Autodesk Inventor part; units mm, degrees
ref_plane "YZ Plane" through (0, 0, 0) normal (1, 0, 0) x (0, 1, 0)
ref_plane "XZ Plane" through (0, 0, 0) normal (0, 1, 0) x (-1, 0, 0)
ref_plane "XY Plane" through (0, 0, 0) normal (0, 0, 1) x (1, 0, 0)
sketch "Szkic1" plane through (0, 0, 0) normal (0, 0, 1) x (1, 0, 0)
  line L0 (-172.0995, -130.735) -> (1627.9005, -130.735)
  line L1 (1627.9005, -130.735) -> (1627.9005, -330.735)
  line L2 (1627.9005, -330.735) -> (-172.0995, -330.735)
  line L3 (-172.0995, -330.735) -> (-172.0995, -130.735)
  dimension "d6" = 1800
  dimension "d7" = 200
extrude "Wyciągnięcie proste1" add sketch "Szkic1" along normal blind 1100
sketch "Szkic2" plane through (-172.0995, -130.735, 0) normal (0, 1, 0) x (1, 0, 0)
  point P0 (172.0995, 0)
sketch "Szkic3" plane through (-172.0995, -130.735, 0) normal (0, 1, 0) x (1, 0, 0)
  line L0 (0, 0) -> (1800, 0)
  line L1 (0, -1100) -> (1800, -1100)
  line L2 (0, 0) -> (200, 0)
  line L3 (200, 0) -> (200, -1100)
  line L4 (200, -1100) -> (0, -1100)
  line L5 (0, -1100) -> (0, 0)
  line L6 (1800, 0) -> (1700, 0)
  line L7 (1700, -1100) -> (1800, -1100)
  line L8 (1334, 0) -> (1134, 0)
  line L9 (1134, 0) -> (1134, -1100)
  line L10 (1134, -1100) -> (1334, -1100)
  line L11 (1334, -1100) -> (1334, 0)
  line L12 (100, 0) -> (100, -1100)
  line L13 (1234, 0) -> (1234, -1100) construction
  point P0 (172.0995, 0)
  point P1 (1134, 0)
  dimension "d10" = 200
  dimension "d15" = 200
  dimension "d21" = 934
extrude "Wyciągnięcie proste2" add sketch "Szkic3" along normal blind 1200 contours L0 L12 L1 L5 | L0 L3 L1 L12 | L0 L11 L1 L9
sketch "Szkic6" plane through (27.9005, -130.735, 1100) normal (1, 0, 0) x (0, 0, -1)
  line L0 (0, 1200) -> (1100, 1200)
  line L1 (550, 1200) -> (550, 0)
  line L2 (1100, 0) -> (0, 0)
  line L3 (0, 0) -> (0, 1200)
  line L4 (0, 600) -> (1100, 600)
  line L5 (1100, 0) -> (1100, 1200)
  circle A0 centre (550, 600) radius 85
  point P0 (1100, 130.735)
  dimension "d23" = 170
extrude "Wyciągnięcie proste4" cut sketch "Szkic6" along normal blind 982 and the other way blind 46 contours A0 L4 L1 | L1 L4 A0 | L4 L1 A0 | L4 A0 L1
sketch "Szkic7" plane through (1161.9005, -130.735, 1100) normal (1, 0, 0) x (0, 0, -1)
  point P0 (1100, 130.735)
sketch "Szkic8" plane through (1161.9005, -130.735, 1100) normal (1, 0, 0) x (0, 0, -1)
  circle A0 centre (550, 600) radius 85
  circle A1 centre (550, 600) radius 132
  point P0 (1100, 130.735)
  dimension "d28" = 264
extrude "Wyciągnięcie proste5" cut sketch "Szkic8" against normal up to surface (152 mm away) contours A0 | A1
sketch "Szkic9" plane through (-172.0995, -330.735, 0) normal (-1, 0, 0) x (0, 0, 1)
  circle A0 centre (550, 800) radius 85
  circle A1 centre (550, 800) radius 132
  point P0 (0, 330.735)
extrude "Wyciągnięcie proste6" cut sketch "Szkic9" against normal up to surface (154 mm away) contours A0 | A1
sketch "Szkic10" plane through (1161.9005, -130.735, 1100) normal (1, 0, 0) x (0, 0, -1)
  line L0 (1100, 1200) -> (0, 1200)
  line L1 (1100, 0) -> (0, 0)
  line L2 (0, -200) -> (0, 1200)
  circle A0 centre (550, 600) radius 250
  line L3 (0, 0) -> (322.7328, 704.1616)
  line L4 (1100, 0) -> (777.2672, 704.1616)
  line L5 (0, 0) -> (0, 1200)
  line L6 (0, 1200) -> (1100, 1200)
  line L7 (1100, -200) -> (1100, 1200)
  line L8 (1100, 1200) -> (1100, 0)
  point P0 (1100, 130.735)
  dimension "d33" = 500
extrude "Wyciągnięcie proste7" cut sketch "Szkic10" against normal through all contours L7 L4 A0 L3 L2 L0
sketch "Szkic11" plane through (-172.0995, -330.735, 0) normal (-1, 0, 0) x (0, 0, 1)
  circle A0 centre (550, 800) radius 132
  circle A1 centre (550, 800) radius 85
  circle A2 centre (550, 800) radius 250
  line L0 (0, 200) -> (1100, 200)
  line L1 (0, 0) -> (1100, 0)
  line L2 (1100, 0) -> (1100, 200)
  line L3 (1100, 200) -> (0, 200)
  line L4 (0, 200) -> (0, 0)
  line L5 (1100, 200) -> (777.2672, 904.1616)
  line L6 (1100, 200) -> (777.2672, 904.1616)
  line L7 (322.7328, 904.1616) -> (0, 200)
  line L8 (0, 200) -> (322.7328, 904.1616)
  point P0 (0, 330.735)
extrude "Wyciągnięcie proste8" add sketch "Szkic11" along normal blind 48 contours A2 | A2 L5 L0 L7 | L2 L1 L4 L0
sketch "Szkic12" plane through (-220.0995, -330.735, 0) normal (-1, 0, 0) x (0, 0, 1)
  point P0 (0, 330.735)
sketch "Szkic13" plane through (-18.0995, 469.265, 550) normal (-1, 0, 0) x (0, 0, 1)
  point P0 (-550, -469.265)
ref_plane "Płaszczyzna konstrukcyjna1" through (-220.0995, -330.735, 0) normal (-1, 0, 0) x (0, 0, 1)
sketch "Szkic14" plane through (-220.0995, -330.735, 0) normal (-1, 0, 0) x (0, 0, 1)
  point P0 (0, 330.735)
sketch "Szkic15" plane through (-220.0995, -330.735, 0) normal (-1, 0, 0) x (0, 0, 1)
  point P0 (0, 330.735)
sketch "Szkic16" plane through (-220.0995, -330.735, 0) normal (-1, 0, 0) x (0, 0, 1)
  circle A0 centre (550, 980) radius 18
  point P0 (0, 330.735)
  dimension "d39" = 36
extrude "Wyciągnięcie proste9" cut sketch "Szkic16" against normal blind 35
sketch "Szkic18" plane through (-220.0995, -330.735, 0) normal (-1, 0, 0) x (0, 0, 1)
  circle A0 centre (550, 620) radius 18
  circle A1 centre (370, 800) radius 18
  point P0 (0, 330.735)
  dimension "d43" = 36
  dimension "d44" = 36
extrude "Wyciągnięcie proste10" cut sketch "Szkic18" against normal blind 35
thread "Gwint1"
thread "Gwint2"
thread "Gwint3"
sketch "Szkic19" plane through (-220.0995, -330.735, 0) normal (-1, 0, 0) x (0, 0, 1)
  circle A0 centre (730, 800) radius 18
  point P0 (0, 330.735)
  dimension "d57" = 36
extrude "Wyciągnięcie proste12" cut sketch "Szkic19" against normal blind 35
thread "Gwint5"
sketch "Szkic20" plane through (27.9005, -130.735, 1100) normal (1, 0, 0) x (0, 0, -1)
  point P0 (1100, 130.735)
sketch "Szkic26" plane through (961.9005, -130.735, 0) normal (-1, 0, 0) x (0, 0, 1)
  circle A0 centre (550, 600) radius 85
  circle A1 centre (550, 600) radius 250
  point P0 (0, 130.735)
extrude "Wyciągnięcie proste15" add sketch "Szkic26" along normal blind 126
sketch "Szkic27" plane through (835.9005, 469.265, 550) normal (-1, 0, 0) x (0, 0, 1)
  circle A0 centre (0, 0) radius 87
  circle A1 centre (0, 0) radius 92
  point P0 (-550, -469.265)
  dimension "d71" = 174
  dimension "d72" = 184
extrude "Wyciągnięcie proste16" cut sketch "Szkic27" against normal blind 8
sketch "Szkic28" plane through (-220.0995, -330.735, 0) normal (-1, 0, 0) x (0, 0, 1)
  point P0 (0, 330.735)
sketch "Szkic29" plane through (1161.9005, -130.735, 1100) normal (1, 0, 0) x (0, 0, -1)
  circle A0 centre (550, 780) radius 18
  circle A1 centre (550, 780) radius 18
  circle A2 centre (730, 600) radius 18
  circle A3 centre (730, 600) radius 18
  circle A4 centre (550, 420) radius 18
  circle A5 centre (550, 420) radius 18
  circle A6 centre (370, 600) radius 18
  circle A7 centre (370, 600) radius 18
  point P0 (1100, 130.735)
  dimension "d75" = 36
  dimension "d76" = 36
  dimension "d77" = 36
  dimension "d78" = 36
extrude "Wyciągnięcie proste17" cut sketch "Szkic29" against normal blind 35
thread "Gwint6"
thread "Gwint7"
thread "Gwint8"
thread "Gwint9"
sketch "Szkic30" plane through (27.9005, -130.735, 1100) normal (1, 0, 0) x (0, 0, -1)
  circle A0 centre (550, 600) radius 250
  point P0 (1100, 130.735)
  dimension "d89" = 500
extrude "Wyciągnięcie proste18" add sketch "Szkic30" along normal blind 126
sketch "Szkic31" plane through (153.9005, 469.265, 550) normal (1, 0, 0) x (0, 0, -1)
  point P0 (550, -469.265)
sketch "Szkic32" plane through (153.9005, 469.265, 550) normal (1, 0, 0) x (0, 0, -1)
  circle A0 centre (0, 0) radius 85
  circle A1 centre (0, 0) radius 85
  point P0 (550, -469.265)
  dimension "d92" = 170
extrude "Wyciągnięcie proste19" cut sketch "Szkic32" against normal blind 400
sketch "Szkic33" plane through (153.9005, 469.265, 550) normal (1, 0, 0) x (0, 0, -1)
  circle A0 centre (0, 0) radius 87
  circle A1 centre (0, 0) radius 92
  point P0 (550, -469.265)
  dimension "d95" = 174
  dimension "d96" = 184
extrude "Wyciągnięcie proste20" cut sketch "Szkic33" against normal blind 8
properties part number "podstawa"
Check sheet for the modelled part. Datum: model origin and axes. Units: mm. A direction names the side the tool comes from. Coordinates: 2 decimals unless noted, no trailing zeros. Loops run counter-clockwise (first coordinate to the right, second up) from the corner with the lowest first, then second, coordinate; pieces in that order, holes last. Notation, with made-up numbers: (33.25, 33.25) -> (76.25, 33.25) arc R18 ccw to (76.25, 44.25) -> close; hole circle Ø7 at (-10.5, -18). An arc over 180 degrees is marked (long way). Answer in a Markdown table with one row per item.
1. Sectioned sample at A-A, the plane y = 24. Record the boundary of the cut face in (x, z), then the cut area to 3 significant figures.
Check values:
| item | result |
|---|---|
| outline | (-220.1, 70.92) -> (27.9, 70.92) -> (27.9, 1029.08) -> (-220.1, 1029.08) -> close; (961.9, 70.92) -> (1161.9, 70.92) -> (1161.9, 1029.08) -> (961.9, 1029.08) -> close |
| area | 429,000 mm2 |
2. Release check for a two-part mould opening along Y. For faces 1 (the face through (149.956, 413.284, 623.008)), 2 (the face through (1161.9, 194, 558)), 3 (the face through (717, -330.735, 542)) record: released by +Y, released by -Y, zero draft, split by the parting line, or undercut.
Check values:
| item | result |
|---|---|
| face 1 | undercut |
| face 2 | zero draft |
| face 3 | released by -Y |
3. Go/stop test with flat-tipped pins: pin 1 (11 mm diameter, centred on y = 645, z = 548, fed in from +X); pin 2 (5 mm diameter, centred on y = 585, z = 595.5, fed in from +X); pin 3 (1.5 mm diameter, centred on x = -6.5, z = 701.5, fed in from +Y). Record where each tip stops, or that it passes through.
Check values:
| item | result |
|---|---|
| pin 1 | stops at x = 1126.9 |
| pin 2 | stops at x = 1009.9 |
| pin 3 | stops at y = 668.7 |
4. Material ranges on line 1 along Y through (x, z) = (-196, 550) (3 decimals); line 2 along Y through (x, z) = (1124.5, 550) (3 decimals); line 3 along X through (y, z) = (529, 696), recorded low to high. Write a range as [from, to].
Check values:
| item | result |
|---|---|
| line 1 | y = [-330.735, 271.265], [307.265, 337.265], [601.265, 631.265], [667.265, 719.265] |
| line 2 | y = [-330.735, 337.265], [601.265, 719.265] |
| line 3 | x = [-220.1, 153.9], [835.9, 1161.9] |
5. Sectioned sample at B-B, the plane z = 499. Give the number of separate pieces and of enclosed holes in the cut face, then the cut area to 3 significant figures.
Check values:
| item | result |
|---|---|
| separate pieces | 3 |
| enclosed holes | 0 |
| area | 738,000 mm2 |
6. Sectioned sample at C-C, the plane x = 1192. Record the boundary of the cut face in (y, z) (3 decimals).
Check values:
| item | result |
|---|---|
| outline | (-330.735, 0) -> (-130.735, 0) -> (-130.735, 1100) -> (-330.735, 1100) -> close |
7. Access from +Z, -Z, +X, -X, +Y, -Y to the whole of each face (thin tool, end or side, straight path). Record for faces 4 (the face through (1086.964, 558.477, 647.289)), 5 (the face through (835.9, 450, 633)), 6 (the face through (-94.4, 216.4, 159.1)), 7 (the face through (-202.844, 462.371, 746.627)), 8 (the face through (839.84, 379.45, 530.06)).
Check values:
| item | result |
|---|---|
| face 4 | +X |
| face 5 | +Z, -Z, +Y |
| face 6 | -Z, +X, -X, +Y |
| face 7 | -X |
| face 8 | none |
